Part model, mm, in its own coordinate system. Give positions to 0.01 mm unless a question says otherwise; leave off trailing zeros. Write each loop counter-clockwise with the first axis right and the second up, starting at its lowest first coordinate (ties: lowest second). Pieces come first, ordered by that corner, then holes. Notation, with made-up numbers: M -18.75,-13 L 8.25,-13 A23 cw 8.25,12 Z; hole C 76,7 d8. An arc over 180 degrees is marked long. Use CSV: the item, a comma, the result in double quotes. Start each with the question number.
Item 1: Pin check, flat tips, straight feed: pin 1 (3.5 mm diameter, centred on x = -104.17, y = -24.57, fed in from +Z); pin 2 (1.5 mm diameter, centred on x = -91.5, y = 21.5, fed in from +Z); pin 3 (4 mm diameter, centred on x = -78.65, y = 61.39, fed in from -Z); pin 4 (2.5 mm diameter, centred on x = -128.17, y = -24.57, fed in from +Z). Stop position of each tip, or through.
Item 2: Drill centre lines: line 1 (X direction, y = 63.5, z = 1.7); line 2 (Y direction, x = -117, z = 1.75); line 3 (Y direction, x = -15, z = 0.65). Where is each one in solid material? Low to high. Write a range as [from, to].
Item 3: Cut at A-A (x = -110.5). List the corners of the cut face in (y, z).
Item 4: Cut at C-C (y = 22.5). List the corners of the cut face in (x, z).
Item 5: Mould opens along Y. For faces 1 (the flat face through (-36, 33, 2.2)), 2 (the flat face through (-106, 52, 1)) say: released by +Y, released by -Y, zero draft, split by the parting line, or undercut.
Item 6: Cut at B-B (z = 1.8). Count the separate pieces of the cut face and the enclosed holes in it, then the cut area to 3 significant figures.
Item 7: Cut at D-D (x = 6.5). List the corners of the cut face in (y, z).
from build123d import *

# Parameters (mm, degrees)
BOSS_EXTRUDE1_DEPTH                            = 2.2
CSK_FOR_M2_5_COUNTERSUNK_FLAT_HEAD_S_2_COUNT   = 2
CSK_FOR_M2_5_COUNTERSUNK_FLAT_HEAD_S_2_PITCH   = 115.901286123
CSK_FOR_M2_5_COUNTERSUNK_FLAT_HEAD_S_3_COUNT   = 2
CSK_FOR_M2_5_COUNTERSUNK_FLAT_HEAD_S_3_PITCH   = 127.813646083
CSK_FOR_M2_5_COUNTERSUNK_FLAT_HEAD_S_4_COUNT   = 2
CSK_FOR_M2_5_COUNTERSUNK_FLAT_HEAD_S_4_PITCH   = 57.15
CSK_FOR_M2_5_COUNTERSUNK_FLAT_HEAD_S_5_A_COUNT = 2
CSK_FOR_M2_5_COUNTERSUNK_FLAT_HEAD_S_5_A_PITCH = 24
CSK_FOR_M2_5_COUNTERSUNK_FLAT_HEAD_S_6_COUNT   = 2
CSK_FOR_M2_5_COUNTERSUNK_FLAT_HEAD_S_6_PITCH   = 114
CSK_FOR_M2_5_COUNTERSUNK_FLAT_HEAD_S_7_COUNT   = 2
CSK_FOR_M2_5_COUNTERSUNK_FLAT_HEAD_S_7_PITCH   = 116.498927034
CUT_EXTRUDE1_DEPTH                             = 161.482952565
CUT_EXTRUDE1_DEPTH_BACK                        = 1.2
SKETCH4_W                                      = 40
SKETCH4_H                                      = 69


with BuildPart() as part:
    # Sketch1 → Boss-Extrude1 (new body)
    with BuildSketch(Plane.XY):
        with BuildLine():
            Line((-129.172572744, -27.567893977), (-103.172572744, -27.567893977))
            ThreePointArc((-103.172572744, -27.567893977), (-101.758359182, -26.98210754), (-101.172572744, -25.567893977))
            Line((-101.172572744, -25.567893977), (-101.172572744, -22.567893977))
            Line((-101.172572744, -22.567893977), (59.877427256, -22.567893977))
            ThreePointArc((59.877427256, -22.567893977), (61.291640818, -21.98210754), (61.877427256, -20.567893977))
            Line((61.877427256, -20.567893977), (61.877427256, 85.432106023))
            ThreePointArc((61.877427256, 85.432106023), (61.291640818, 86.846319585), (59.877427256, 87.432106023))
            Line((59.877427256, 87.432106023), (-101.172572744, 87.432106023))
            Line((-101.172572744, 87.432106023), (-101.172572744, 90.432106023))
            ThreePointArc((-101.172572744, 90.432106023), (-101.758359182, 91.846319585), (-103.172572744, 92.432106023))
            Line((-103.172572744, 92.432106023), (-129.172572744, 92.432106023))
            ThreePointArc((-129.172572744, 92.432106023), (-130.586786306, 91.846319585), (-131.172572744, 90.432106023))
            Line((-131.172572744, 90.432106023), (-131.172572744, -25.567893977))
            ThreePointArc((-131.172572744, -25.567893977), (-130.586786306, -26.98210754), (-129.172572744, -27.567893977))
        make_face()
    extrude(amount=BOSS_EXTRUDE1_DEPTH)

    # Sketch2 → CSK for M2.5 Countersunk Flat Head Screw (revolve, cut)
    with BuildSketch(Plane(origin=(-78.647572744, 61.391992259, 0), x_dir=(0, 1, 0), z_dir=(1, 0, 0))):
        Polygon((0, 0), (0, 2.2), (1.45, 2.2), (1.45, 1.3), (2.75, 0), align=None)
    csk_for_m2_5_countersunk_flat_head_screw = revolve(axis=Axis((-78.647572744, 61.391992259, -6.35), (0, 0, 1)), mode=Mode.SUBTRACT)

    # CSK for M2.5 Countersunk Flat Head S 2: CSK for M2.5 Countersunk Flat Head Screw ×2
    with Locations(*[Vector(0.9863997529632768, -0.1643640086940774, 0) * (i * CSK_FOR_M2_5_COUNTERSUNK_FLAT_HEAD_S_2_PITCH) for i in range(1, CSK_FOR_M2_5_COUNTERSUNK_FLAT_HEAD_S_2_COUNT)]):
        add(csk_for_m2_5_countersunk_flat_head_screw, mode=Mode.SUBTRACT)

    # CSK for M2.5 Countersunk Flat Head S 3: CSK for M2.5 Countersunk Flat Head Screw ×2
    with Locations(*[Vector(0.8944663070316109, -0.447135354881754, 0) * (i * CSK_FOR_M2_5_COUNTERSUNK_FLAT_HEAD_S_3_PITCH) for i in range(1, CSK_FOR_M2_5_COUNTERSUNK_FLAT_HEAD_S_3_COUNT)]):
        add(csk_for_m2_5_countersunk_flat_head_screw, mode=Mode.SUBTRACT)

    # CSK for M2.5 Countersunk Flat Head S 4: CSK for M2.5 Countersunk Flat Head Screw ×2
    with Locations(*[(0, -i * CSK_FOR_M2_5_COUNTERSUNK_FLAT_HEAD_S_4_PITCH, 0) for i in range(1, CSK_FOR_M2_5_COUNTERSUNK_FLAT_HEAD_S_4_COUNT)]):
        add(csk_for_m2_5_countersunk_flat_head_screw, mode=Mode.SUBTRACT)

    # Sketch3 → CSK for M2.5 Countersunk Flat Head S 5 (revolve, cut)
    with BuildSketch(Plane(origin=(-104.172572744, 89.432106023, 0), x_dir=(0, 1, 0), z_dir=(1, 0, 0))):
        Polygon((0, 0), (0, 2.2), (1.45, 2.2), (1.45, 1.3), (2.75, 0), align=None)
    csk_for_m2_5_countersunk_flat_head_s_5 = revolve(axis=Axis((-104.172572744, 89.432106023, -6.35), (0, 0, 1)), mode=Mode.SUBTRACT)

    # CSK for M2.5 Countersunk Flat Head S 5 a: CSK for M2.5 Countersunk Flat Head S 5 ×2
    with Locations(*[(-i * CSK_FOR_M2_5_COUNTERSUNK_FLAT_HEAD_S_5_A_PITCH, 0, 0) for i in range(1, CSK_FOR_M2_5_COUNTERSUNK_FLAT_HEAD_S_5_A_COUNT)]):
        add(csk_for_m2_5_countersunk_flat_head_s_5, mode=Mode.SUBTRACT)

    # CSK for M2.5 Countersunk Flat Head S 6: CSK for M2.5 Countersunk Flat Head S 5 ×2
    with Locations(*[(0, -i * CSK_FOR_M2_5_COUNTERSUNK_FLAT_HEAD_S_6_PITCH, 0) for i in range(1, CSK_FOR_M2_5_COUNTERSUNK_FLAT_HEAD_S_6_COUNT)]):
        add(csk_for_m2_5_countersunk_flat_head_s_5, mode=Mode.SUBTRACT)

    # CSK for M2.5 Countersunk Flat Head S 7: CSK for M2.5 Countersunk Flat Head S 5 ×2
    with Locations(*[Vector(-0.20601048104984218, -0.9785497849867489, 0) * (i * CSK_FOR_M2_5_COUNTERSUNK_FLAT_HEAD_S_7_PITCH) for i in range(1, CSK_FOR_M2_5_COUNTERSUNK_FLAT_HEAD_S_7_COUNT)]):
        add(csk_for_m2_5_countersunk_flat_head_s_5, mode=Mode.SUBTRACT)

    # Sketch4 → Cut-Extrude1 (cut, two sides: drawn at the far end of the back side and taken through both)
    with BuildSketch(Plane.XY.offset(2.2).offset(-CUT_EXTRUDE1_DEPTH_BACK)):
        with Locations((-106.172572744, 51.432106023)):
            Rectangle(SKETCH4_W, SKETCH4_H)
    extrude(amount=CUT_EXTRUDE1_DEPTH + CUT_EXTRUDE1_DEPTH_BACK, mode=Mode.SUBTRACT)


solid = part.part
Worked answers:
1,pin 1,"stops at z = 2.2"
1,pin 2,"stops at z = 1"
1,pin 3,"stops at z = 0.75"
1,pin 4,"passes through"
2,line 1,"x = [-131.17, -126.17], [-86.17, 61.88]"
2,line 2,"y = [-27.57, 16.93], [85.93, 92.43]"
2,line 3,"y = [-22.57, 87.43]"
3,outline,"M -27.57,0 L 92.43,0 L 92.43,2.2 L 85.93,2.2 L 85.93,1 L 16.93,1 L 16.93,2.2 L -27.57,2.2 Z"
4,outline,"M -131.17,0 L 61.88,0 L 61.88,2.2 L -86.17,2.2 L -86.17,1 L -126.17,1 L -126.17,2.2 L -131.17,2.2 Z"
5,face 1,"zero draft"
5,face 2,"undercut"
6,separate pieces,"1"
6,enclosed holes,"9"
6,area,"18,700 mm^2"
7,outline,"M -22.57,0 L 87.43,0 L 87.43,2.2 L -22.57,2.2 Z"
